Check sheet for the modelled part. Datum: model origin and axes. Units: mm. A direction names the side the tool comes from. Round coordinates to 2 decimals unless told otherwise and drop trailing zeros. Loops run counter-clockwise (first coordinate to the right, second up) from the corner with the lowest first, then second, coordinate; pieces in that order, holes last. Notation, with made-up numbers: (-22.5, 11.5) - (23.5, 11.5) arc R29 cw to (23.5, 42.5) - close; hole circle Ø4 at (18, -31.5). An arc over 180 degrees is marked (long way). Answer in a Markdown table with one row per item. Add a question column.
(1) Cross-section at B-B on y = 46.5. Count the separate pieces of the cut face and the enclosed holes in it, then the cut area to 3 significant figures.
(2) Mould release check, pull along Z, two halves, no side actions. Record for faces 6 (the flat face through (-7.8, 14.3, -13.4)), 7 (the flat face through (21, 6, 2)), 8 (the flat face through (21, 0, -10)): +Z half, -Z half, draft (parallel to the pull), parting line (faces both ways), or undercut.
(3) Gauge pin test, flat ends, axial feed: pin 1 (8 mm diameter, centred on x = 9.5, z = -16.5, fed in from +Y); pin 2 (12 mm diameter, centred on x = 31, y = 42, fed in from -Z); pin 3 (6 mm diameter, centred on x = 27.5, z = -15, fed in from +Y). Record the tip position at first contact, or that the pin passes through.
(4) Thickness scan on line 1 along X through (y, z) = (7.75, -15.2); line 2 along X through (y, z) = (25, -16.5); line 3 along Z through (x, y) = (-4, 21). Record the ranges inside material, lowest first.
(5) Access from +Z, -Z, +X, -X, +Y, -Y to the whole of each face (thin tool, end or side, straight path). Record for faces 1 (the flat face through (22, 27.9, 1)), 2 (the cylindrical face through (2.27, 47.97, -27.6)), 3 (the cylindrical face through (26.814, 31.852, -22.925)), 4 (the flat face through (-4, 14, -13.2)), 5 (the flat face through (-3, 38, 6)).
(6) Cross-section at A-A on z = -15.2. Enter the section's corners in (x, y), then the cut area to 3 significant figures.
from build123d import *

# Parameters (mm, degrees)
SKETCH1_W               = 56
SKETCH1_H               = 24.4
SKETCH1_W_2             = 40.4
SKETCH1_H_2             = 20.4
BOSS_EXTRUDE1_DEPTH     = 27.9
SKETCH2_W               = 56
SKETCH2_H               = 24.4
BOSS_EXTRUDE2_DEPTH     = 1
BOSS_EXTRUDE3_DEPTH     = 56
SKETCH4_R               = 1.7
CUT_EXTRUDE1_DEPTH      = 79.056453929
CUT_EXTRUDE2_START      = -10
SKETCH5_R               = 3
CUT_EXTRUDE2_DEPTH      = 69.056453929
CHAMFER1_SIZE           = 10
CHAMFER1_SIZE2          = 5.773502692
CHAMFER2_SIZE           = 10
CHAMFER2_SIZE2          = 5.773502692
CHAMFER3_SIZE           = 10
CHAMFER3_SIZE2          = 5.773502692
CHAMFER4_SIZE           = 10
CHAMFER4_SIZE2          = 5.773502692
SKETCH6_W               = 7.8
SKETCH6_H               = 6
CUT_EXTRUDE3_DEPTH      = 27.9
SKETCH7_R               = 1.1
CUT_EXTRUDE4_DEPTH      = 30
CUT_EXTRUDE5_DEPTH      = 79.056453929
CUT_EXTRUDE6_DEPTH      = 79.151199776
CUT_EXTRUDE6_DEPTH_BACK = 79.151199776


with BuildPart() as part:
    # Sketch1 → Boss-Extrude1 (new body)
    with BuildSketch(Plane(origin=(0, 0, 0), x_dir=(1, 0, 0), z_dir=(0, 1, 0))):
        with Locations((20.2, 10.2)):
            Rectangle(SKETCH1_W, SKETCH1_H)
        with Locations((20.2, 10.2)):
            Rectangle(SKETCH1_W_2, SKETCH1_H_2, mode=Mode.SUBTRACT)
    extrude(amount=BOSS_EXTRUDE1_DEPTH)

    # Sketch2 → Boss-Extrude2 (add)
    with BuildSketch(Plane(origin=(0, 0, 0), x_dir=(-1, 0, 0), z_dir=(0, -1, 0))):
        with Locations((-20.2, 10.2)):
            Rectangle(SKETCH2_W, SKETCH2_H)
    extrude(amount=BOSS_EXTRUDE2_DEPTH)

    # Sketch3 → Boss-Extrude3 (add)
    with BuildSketch(Plane(origin=(48.2, 0, 0), x_dir=(0, 0, -1), z_dir=(1, 0, 0))):
        Polygon((22.4, 12.9), (29.4, 27.9), (29.4, 52.9), (22.4, 52.9), align=None)
    boss_extrude3 = extrude(amount=-BOSS_EXTRUDE3_DEPTH)

    # Sketch4 → Cut-Extrude1 (cut, through all)
    with BuildSketch(Plane(origin=(0, 52.9, 0), x_dir=(1, 0, 0), z_dir=(0, 1, 0))):
        with Locations(Location((2.2, 25.9, 0), (0, 0, 270))):
            Circle(SKETCH4_R)
        with Locations(Location((27.2, 25.9, 0), (0, 0, 270))):
            Circle(SKETCH4_R)
    cut_extrude1 = extrude(amount=-CUT_EXTRUDE1_DEPTH, mode=Mode.SUBTRACT)

    # Sketch5 → Cut-Extrude2 (cut, through all)
    with BuildSketch(Plane(origin=(0, 52.9, 0), x_dir=(1, 0, 0), z_dir=(0, 1, 0)).offset(CUT_EXTRUDE2_START)):
        with Locations(Location((2.2, 25.9, 0), (0, 0, 270))):
            Circle(SKETCH5_R)
        with Locations(Location((27.2, 25.9, 0), (0, 0, 270))):
            Circle(SKETCH5_R)
    cut_extrude2 = extrude(amount=-CUT_EXTRUDE2_DEPTH, mode=Mode.SUBTRACT)

    # Mirror1: Boss-Extrude3, Cut-Extrude1, Cut-Extrude2 across plane
    add(boss_extrude3.mirror(Plane.XY.offset(-10.2)))
    add(cut_extrude1.mirror(Plane.XY.offset(-10.2)), mode=Mode.SUBTRACT)
    add(cut_extrude2.mirror(Plane.XY.offset(-10.2)), mode=Mode.SUBTRACT)

    # Chamfer1
    chamfer1_edges = [part.edges().sort_by_distance(p)[0] for p in [
        (-7.8, 40.4, -29.4),
    ]]
    chamfer1_side = [part.faces().sort_by_distance(p)[0] for p in [
        (20.2, 40.4, -29.4),
    ]]
    chamfer(chamfer1_edges, length=CHAMFER1_SIZE, length2=CHAMFER1_SIZE2, reference=chamfer1_side[0])

    # Chamfer2
    chamfer2_edges = [part.edges().sort_by_distance(p)[0] for p in [
        (48.2, 40.4, -29.4),
    ]]
    chamfer2_side = [part.faces().sort_by_distance(p)[0] for p in [
        (25.2, 40.4, -29.4),
    ]]
    chamfer(chamfer2_edges, length=CHAMFER2_SIZE, length2=CHAMFER2_SIZE2, reference=chamfer2_side[0])

    # Chamfer3
    chamfer3_edges = [part.edges().sort_by_distance(p)[0] for p in [
        (-7.8, 40.4, 9),
    ]]
    chamfer3_side = [part.faces().sort_by_distance(p)[0] for p in [
        (20.2, 40.4, 9),
    ]]
    chamfer(chamfer3_edges, length=CHAMFER3_SIZE, length2=CHAMFER3_SIZE2, reference=chamfer3_side[0])

    # Chamfer4
    chamfer4_edges = [part.edges().sort_by_distance(p)[0] for p in [
        (48.2, 40.4, 9),
    ]]
    chamfer4_side = [part.faces().sort_by_distance(p)[0] for p in [
        (25.2, 40.4, 9),
    ]]
    chamfer(chamfer4_edges, length=CHAMFER4_SIZE, length2=CHAMFER4_SIZE2, reference=chamfer4_side[0])

    # Sketch6 → Cut-Extrude3 (cut)
    with BuildSketch(Plane(origin=(0, 27.9, 0), x_dir=(1, 0, 0), z_dir=(0, 1, 0))):
        with Locations((-3.9, 10.2)):
            Rectangle(SKETCH6_W, SKETCH6_H)
    extrude(amount=-CUT_EXTRUDE3_DEPTH, mode=Mode.SUBTRACT)

    # Sketch7 → Cut-Extrude4 (cut)
    with BuildSketch(Plane(origin=(0, 27.9, 0), x_dir=(1, 0, 0), z_dir=(0, 1, 0))):
        with Locations(Location((-4.3, 15.2, 0), (0, 0, 270))):
            Circle(SKETCH7_R)
        with Locations(Location((-4.3, 5.2, 0), (0, 0, 270))):
            Circle(SKETCH7_R)
        with Locations(Location((44.7, 15.2, 0), (0, 0, 270))):
            Circle(SKETCH7_R)
        with Locations(Location((44.7, 5.2, 0), (0, 0, 270))):
            Circle(SKETCH7_R)
    extrude(amount=-CUT_EXTRUDE4_DEPTH, mode=Mode.SUBTRACT)

    # Sketch8 → Cut-Extrude5 (cut, symmetric)
    with BuildSketch(Plane(origin=(0, 52.9, 0), x_dir=(1, 0, 0), z_dir=(0, 1, 0))):
        with BuildLine():
            add(Edge.make_bspline(
                [(2.2, 29.4), (38.687561205, 29.118506407), (48.2, 23.626497308)],
                knots=[0, 0, 0, 1, 1, 1], degree=2))
            Line((48.2, 23.626497308), (38.2, 29.4))
            Line((38.2, 29.4), (2.2, 29.4))
        make_face()
    cut_extrude5 = extrude(amount=CUT_EXTRUDE5_DEPTH, both=True, mode=Mode.SUBTRACT)

    # Mirror2: Cut-Extrude5 across plane
    add(cut_extrude5.mirror(Plane.XY.offset(-10.2)), mode=Mode.SUBTRACT)

    # Sketch9 → Cut-Extrude6 (cut, two sides: drawn at the far end of the back side and taken through both)
    with BuildSketch(Plane.XY.offset(2).offset(-CUT_EXTRUDE6_DEPTH_BACK)):
        with BuildLine():
            Line((33.2, 52.9), (48.2, 52.9))
            Line((48.2, 52.9), (48.2, 42.9))
            ThreePointArc((48.2, 42.9), (41.270707085, 48.756060628), (33.2, 52.9))
        make_face()
    extrude(amount=CUT_EXTRUDE6_DEPTH + CUT_EXTRUDE6_DEPTH_BACK, mode=Mode.SUBTRACT)


solid = part.part
Answers:
| question | item | result |
|---|---|---|
| 1 | separate pieces | 2 |
| 1 | enclosed holes | 4 |
| 1 | area | 540 mm^2 |
| 2 | face 6 | draft |
| 2 | face 7 | +Z half |
| 2 | face 8 | undercut |
| 3 | pin 1 | stops at y = 27.9 |
| 3 | pin 2 | stops at z = -28.52 |
| 3 | pin 3 | stops at y = 0 |
| 4 | line 1 | x = -7.8 to -5.4, -3.2 to 0, 40.4 to 43.6, 45.8 to 48.2 |
| 4 | line 2 | x = -7.8 to 0, 40.4 to 48.2 |
| 4 | line 3 | z = -25.82 to -16.26, -14.14 to -13.2, -7.2 to -6.26, -4.14 to 5.42 |
| 5 | face 1 | +X, -X, +Y |
| 5 | face 2 | +Y, -Y |
| 5 | face 3 | -Y |
| 5 | face 4 | -X, +Y |
| 5 | face 5 | +Z, -X, +Y, -Y |
| 6 | outline | (-7.8, -1) - (-5.4, -1) - (-5.4, 27.9) - (-7.8, 27.9) - close; (-3.2, -1) - (43.6, -1) - (43.6, 27.9) - (40.4, 27.9) - (40.4, 0) - (0, 0) - (0, 27.9) - (-3.2, 27.9) - close; (45.8, -1) - (48.2, -1) - (48.2, 27.9) - (45.8, 27.9) - close |
| 6 | area | 364 mm^2 |
